Check sheet for the modelled part. Datum: model origin and axes. Units: mm. A direction names the side the tool comes from. Give positions to 0.01 mm unless a question says otherwise; leave off trailing zeros. Order: outer loops, then holes, each group sorted by start corner. A loop starts at its lowest first (then second) coordinate and runs counter-clockwise, first axis right, second up.
Item 1: Sectioned sample at B-B on x = -22.5. Record the boundary of the cut face in (y, z), and give its area (3 significant figures).
Item 2: Access from +Z, -Z, +X, -X, +Y, -Y to the whole of each face (thin tool, end or side, straight path). Record for faces 5 (the flat face through (-22, 3.5, -26)), 6 (the flat face through (24, -16.5, -26)), 7 (the flat face through (0, -2, -24.5)).
Item 3: Gauge pin test, flat ends, axial feed: P1, Ø2, axis at x = 6.5, y = -9, coming from the -Z side; P2, Ø8, axis at x = 2, z = -1.5, coming from the -Y side; P3, Ø8.5, axis at x = 5, y = -8, coming from the +Z side; P4, Ø2, axis at x = -0.5, y = 11.5, coming from the +Z side. Record the tip position at first contact, or that the pin passes through.
Item 4: Material ranges on line 1 along Y through (x, z) = (16, -7.5); line 2 along Z through (x, y) = (-24, -8); line 3 along Z through (x, y) = (22, 13), recorded low to high.
Item 5: Sectioned sample at D-D on x = 19.5. Record the boundary of the cut face in (y, z), and give its area (3 significant figures).
Item 6: Release check for a two-part mould opening along X. For faces 1 (the cylindrical face through (0.42, 15.9, -26.93)), 2 (the flat face through (23.6, -4, -26)), 3 (the flat face through (-30, 15, -8)), 4 (the flat face through (30, 15, -8)) record: released by +X, released by -X, zero draft, split by the parting line, or undercut.
Item 7: Sectioned sample at C-C on z = 13. Record the boundary of the cut face in (x, y).
Item 8: Sectioned sample at A-A on y = -5. Record the boundary of the cut face in (x, z).
from build123d import *

# Parameters (mm, degrees)
F1_DEPTH = 30
F2_W     = 3.2
F2_H     = 15
F3_DEPTH = 25
F5_DEPTH = 25
F6_R     = 2


with BuildPart() as f1:
    # F0 (on Right) → F1 (new body, symmetric)
    with BuildSketch(Plane.YZ):
        Polygon((-16.5, -24.5), (-16.5, -27.5), (16.5, -27.5), (16.5, 27.5), (13.5, 27.5), (13.5, -24.5), align=None)
    extrude(amount=F1_DEPTH, both=True)

    # F2 (on face) → F3 (cut)
    with BuildSketch(Plane(origin=(0, 0, -27.5), x_dir=(1, 0, 0), z_dir=(0, 0, -1))):
        with Locations((22, 4)):
            Rectangle(F2_W, F2_H)
        with Locations((-22, 4)):
            Rectangle(F2_W, F2_H)
    extrude(amount=-F3_DEPTH, mode=Mode.SUBTRACT)

    # F4 (on face) → F5 (cut)
    with BuildSketch(Plane(origin=(0, 0, -27.5), x_dir=(1, 0, 0), z_dir=(0, 0, -1))):
        with BuildLine():
            add(Edge.make_bspline(
                [(19.5, 23.5), (19.5, 50.3467875173), (-9.75, 36.9233937587), (-39, 23.5), (-9.75, 10.0766062413), (19.5, -3.3467875173), (19.5, 23.5)],
                knots=[0, 0, 0, 2.0943951024, 2.0943951024, 4.1887902048, 4.1887902048, 6.2831853072, 6.2831853072, 6.2831853072], degree=2, weights=[1, 0.5, 1, 0.5, 1, 0.5, 1]))
        make_face()
    extrude(amount=-F5_DEPTH, mode=Mode.SUBTRACT)

    # F6
    f6_edges = [f1.edges().sort_by_distance(p)[0] for p in [
        (0, 13.5, -24.5),
        (0, 16.5, -27.5),
    ]]
    fillet(f6_edges, radius=F6_R)


solid = f1.part
Report:
1. outline: (-16.5, -27.5) - (-11.5, -27.5) - (-11.5, -24.5) - (-16.5, -24.5) - close; (3.5, -27.5) - (14.5, -27.5) arc R2 ccw to (16.5, -25.5) - (16.5, 27.5) - (13.5, 27.5) - (13.5, -22.5) arc R2 cw to (11.5, -24.5) - (3.5, -24.5) - close
1. area: 210 mm2
2. face 5: +Z, -Z
2. face 6: +Z, -Z, +X, -X, -Y
2. face 7: +Z, +X, -X, -Y
3. P1: stops at z = -27.5
3. P2: stops at y = 13.5
3. P3: stops at z = -24.5
3. P4: stops at z = -24.23
4. line 1: y = 13.5 to 16.5
4. line 2: z = -27.5 to -24.5
4. line 3: z = -27.5 to -23.82
5. outline: (-16.5, -27.5) - (14.5, -27.5) arc R2 ccw to (16.5, -25.5) - (16.5, 27.5) - (13.5, 27.5) - (13.5, -22.5) arc R2 cw to (11.5, -24.5) - (-16.5, -24.5) - close
5. area: 255 mm2
6. face 1: zero draft
6. face 2: undercut
6. face 3: released by -X
6. face 4: released by +X
7. outline: (-30, 13.5) - (30, 13.5) - (30, 16.5) - (-30, 16.5) - close
8. outline: (-30, -27.5) - (-23.6, -27.5) - (-23.6, -24.5) - (-30, -24.5) - close; (-20.4, -27.5) - (20.4, -27.5) - (20.4, -24.5) - (-20.4, -24.5) - close; (23.6, -27.5) - (30, -27.5) - (30, -24.5) - (23.6, -24.5) - close
